Geometry check sheet. Reference: the model listing, model coordinates, mm. Face numbers are marked on the shaded views. A direction names the side the tool comes from. Round coordinates to 2 decimals unless told otherwise and drop trailing zeros. Loops run counter-clockwise (first coordinate to the right, second up) from the corner with the lowest first, then second, coordinate; pieces in that order, holes last. Notation, with made-up numbers: (49, 44) - (65, 44) arc R9 ccw to (65, 56) - close; hole circle Ø4 at (31, 61.25). An arc over 180 degrees is marked (long way). Write item = value, one per line.
Autodesk Inventor part; units mm, degrees
ref_plane "Plano de trabajo3" through (0, 0, 6) normal (0, 0, 1) x (1, 0, 0)
ref_plane "Plano de trabajo1" through (15, 0, 0) normal (1, 0, 0) x (0, 1, 0)
ref_plane "Plano de trabajo2" through (0, 0, 7.5) normal (0, 0, 1) x (1, 0, 0)
sketch "Boceto9" plane through (0, 0, 0) normal (0, 1, 0) x (-1, 0, 0)
  circle A0 centre (0, 0) radius 6
  circle A1 centre (0, 0) radius 2.975
  dimension "d34" = 12
  dimension "d35" = 5.95
extrude "Extrusión9" add sketch "Boceto9" along normal blind 8
sketch "Boceto10" plane through (0, 0, 0) normal (0, -1, 0) x (1, 0, 0)
  circle A0 centre (0, 0) radius 6
  circle A1 centre (0, 0) radius 2.975
  circle A2 centre (0, 0) radius 5
  dimension "d38" = 1
extrude "Extrusión10" add sketch "Boceto10" along normal blind 5 contours A2
sketch "Boceto11" plane through (0, 0, 0) normal (0, -1, 0) x (1, 0, 0)
  circle A0 centre (0, 0) radius 2.975
extrude "Extrusión11" add sketch "Boceto11" along normal blind 2
sketch "Boceto12" plane through (0, -2, 0) normal (0, -1, 0) x (1, 0, 0)
  circle A0 centre (0, 0) radius 2.5
  circle A1 centre (0, 0) radius 2.975
  dimension "d43" = 5
extrude "Extrusión12" add sketch "Boceto12" along normal blind 3
sketch "Boceto13" plane through (0, -5, 0) normal (0, -1, 0) x (1, 0, 0)
  circle A0 centre (0, 0) radius 4
  circle A1 centre (0, 0) radius 5
  dimension "d46" = 8
extrude "Extrusión13" cut sketch "Boceto13" against normal blind 5
chamfer "Chaflán4" distance 0.25 angle 45 1 edges at (-4, -5, 0)
fillet "Empalme2" radius 0.5 1 edges at (-4, 0, 0)
chamfer "Chaflán5" distance 0.5 angle 45 2 edges at (6, 0, 0) (6, 8, 0)
chamfer "Chaflán6" distance 0.5 angle 45 1 edges at (2.975, 8, 0)
ref_plane "Plano de trabajo3" through (0, 0, 6) normal (0, 0, 1) x (1, 0, 0)
sketch "Boceto14" plane through (0, 0, 6) normal (0, 0, 1) x (1, 0, 0)
  line L0 (-6, 0.5) -> (6, 0.5)
  line L1 (6, 7.5) -> (-6, 7.5)
  line L2 (0, 0.5) -> (0, 7.5) construction
  circle A0 centre (0, 4) radius 1.5
  point P0 (0, 0)
  dimension "d60" = 3
extrude "Extrusión14" cut sketch "Boceto14" against normal blind 4
sketch "Boceto1" plane through (0, 0, 0) normal (0, 1, 0) x (-1, 0, 0)
  circle A0 centre (0, 0) radius 15
  dimension "d0" = 30
sketch "Boceto2" plane through (0, 10, 0) normal (0, 1, 0) x (1, 0, 0)
  circle A0 centre (0, 0) radius 2.5
  dimension "d3" = 5
sketch "Boceto3" plane through (0, 0, 0) normal (0, -1, 0) x (1, 0, 0)
  circle A0 centre (0, 0) radius 7.5
  dimension "d6" = 15
sketch "Boceto4" plane through (0, -10, 0) normal (0, -1, 0) x (1, 0, 0)
  circle A0 centre (0, 0) radius 2.975
  dimension "d9" = 5.95
sketch "Boceto6" plane through (0, -10, 0) normal (0, -1, 0) x (1, 0, 0)
  circle A0 centre (0, 0) radius 2.975
  circle A1 centre (0, 0) radius 7.5
sketch "Boceto8" plane through (0, 0, 7.5) normal (0, 0, 1) x (1, 0, 0)
  line L0 (-7.5, -14) -> (7.5, -14)
  line L1 (7.5, -2) -> (-7.5, -2)
  line L2 (7.5, -2) -> (7.5, -14)
  line L3 (-7.5, -2) -> (-7.5, -14)
  line L4 (7.5, -8) -> (-7.5, -8) construction
  circle A0 centre (0, -8) radius 1.5
  point P0 (0, 0)
  dimension "d31" = 3
sketch "Boceto7" plane through (15, 0, 0) normal (1, 0, 0) x (0, 1, 0)
  line L0 (1, 15) -> (1, -15)
  line L1 (14, -15) -> (14, 15)
  line L2 (1, -15) -> (10, -15)
  line L3 (1, 15) -> (10, 15)
  line L4 (7.5, 15) -> (7.5, -15) construction
  circle A0 centre (7.5, 0) radius 1.5
  point P0 (0, 0)
  dimension "d27" = 3
properties part number "Acople_EJE" material "Acero, aleación"
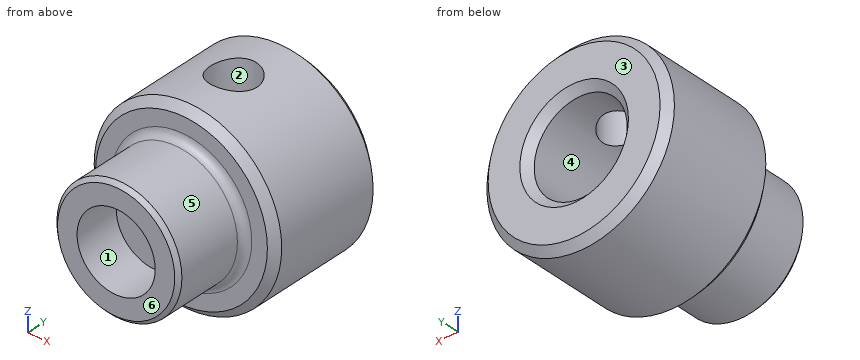
(1) Gauge pin test, flat ends, axial feed: pin 1 (6.5 mm diameter, centred on x = 0, z = 0, fed in from +Y) (3 decimals); pin 2 (3.5 mm diameter, centred on x = 0, z = 0, fed in from +Y). Record the tip position at first contact, or that the pin passes through.
Answers follow:
pin_1 = 7.775
pin_2 = 0
(2) Section check C-C (y = -2.5). Enter the section's corners in (x, z).
Answers follow:
outline = circle Ø8 at (0, 0); hole circle Ø5 at (0, 0)
(3) Section check B-B (z = 0). Enter the section's corners in (x, y) (3 decimals), then the cut area to 3 significant figures.
Answers follow:
outline = (-6, 0.5) - (-5.5, 0) - (-4.5, 0) arc R0.5 cw to (-4, -0.5) - (-4, -4.75) - (-3.75, -5) - (-2.5, -5) - (-2.5, -2) - (2.5, -2) - (2.5, -5) - (3.75, -5) - (4, -4.75) - (4, -0.5) arc R0.5 cw to (4.5, 0) - (5.5, 0) - (6, 0.5) - (6, 7.5) - (5.5, 8) - (3.475, 8) - (2.975, 7.5) - (2.975, 0) - (-2.975, 0) - (-2.975, 7.5) - (-3.475, 8) - (-5.5, 8) - (-6, 7.5) - close
area = 72.7 mm²
(4) Set-up check for the marked faces 1, 2 and 3: record each of +Z, -Z, +X, -X, +Y, -Y from which the full face is reachable in a straight line by a thin tool's end or side.
Answers follow:
face_1 = -Y
face_2 = +Z
face_3 = +Z, -Z, +X, -X, +Y
(5) Section check D-D (y = 1.25). Enter the section's corners in (x, z) (3 decimals), then the cut area to 3 significant figures.
Answers follow:
outline = circle Ø12 at (0, 0); hole circle Ø5.95 at (0, 0)
area = 85.3 mm²
(6) Mould release check, pull along X, two halves, no side actions. Record for the marked faces 4, 5 and 6: pulls with the +X half, pulls with the -X half, needs draft (parallel to the pull), parting line crosses it, or undercut.
Answers follow:
face_4 = undercut
face_5 = parting line crosses it
face_6 = needs draft
(7) Scan lines: L1, parallel to Z at x = 0, y = -3.55; L2, parallel to Y at x = 0, z = 4.7; L3, parallel to Y at x = -3.75, z = 4. Record each from-to range of solid material in increasing order. Write a range as [from, to].
Answers follow:
L1 = [-4, -2.5], [2.5, 4]
L2 = [0, 2.5], [5.5, 8]
L3 = [0, 8]
